```python
from build123d import *

# Parameters (mm, degrees)
F1_DEPTH = 5
F2_W     = 25
F2_H     = 5
F3_DEPTH = 15
F4_F1_R  = 5
F4_F2_R  = 4.9999


# Not quite as in the source:
# - a fillet or chamfer is up to 0.001 mm smaller than in the source, because OpenCascade refuses the exact size


with BuildPart() as f1:
    # F0 (on Front) → F1 (new body)
    with BuildSketch(Plane.XZ):
        with BuildLine():
            Line((-12.5, -22.5), (12.5, -22.5))
            Line((12.5, -22.5), (12.5, 22.5))
            Line((12.5, 22.5), (7.6, 22.5))
            ThreePointArc((7.6, 22.5), (0, 14.9), (-7.6, 22.5))
            Line((-7.6, 22.5), (-12.5, 22.5))
            Line((-12.5, 22.5), (-12.5, -22.5))
        make_face()
    extrude(amount=F1_DEPTH)

    # F2 (on face) → F3 (join)
    with BuildSketch(Plane.XZ.offset(5)):
        with Locations((0, -20)):
            Rectangle(F2_W, F2_H)
    extrude(amount=F3_DEPTH)

    # F4: fillet of radius 5 on 4 edges, made by hand

    # F4_f1
    f4_f1_edges = [f1.edges().sort_by_distance(p)[0] for p in [
        (0, -5, -17.5),
    ]]
    fillet(f4_f1_edges, radius=F4_F1_R)

    # F4_f2 (radius 5 in the source; OpenCascade refuses exactly that, so slightly less here)
    f4_f2_edges = [f1.edges().sort_by_distance(p)[0] for p in [
        (12.5, -15, -17.5),
        (-12.5, -15, -17.5),
        (0, -20, -17.5),
        (-12.5, -6.4644660941, -16.0355339059),
        (12.5, -6.4644660941, -16.0355339059),
    ]]
    fillet(f4_f2_edges, radius=F4_F2_R)


solid = f1.part
```
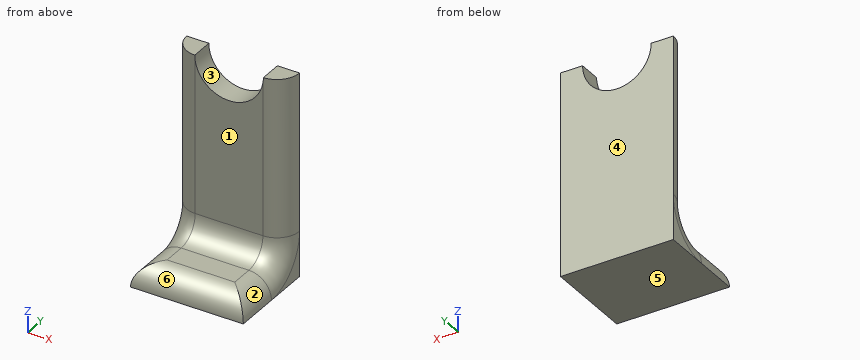
Geometry check sheet. Reference: the model listing, model coordinates, mm. Face numbers are marked on the shaded views. A direction names the side the tool comes from. Coordinates: 2 decimals unless noted, no trailing zeros. Answer in a Markdown table with one row per item. Add a question column.
1. Gauge pin test, flat ends, axial feed: pin 1 Ø5.5 at (x, y) = (2.5, -12) entering from +Z; pin 2 Ø6 at (x, z) = (-10, -8.5) entering from -Y; pin 3 Ø5 at (x, z) = (-9, -12.5) entering from -Y; pin 4 Ø2 at (x, z) = (3, -5.5) entering from +Y. Record the tip position at first contact, or that the pin passes through.
2. Draft check along Y on the marked faces 4, 5 and 6. Enter one of: +Y half, -Y half, draft (parallel to the pull), parting line (faces both ways), or undercut.
3. Access from +Z, -Z, +X, -X, +Y, -Y to the whole of each face (thin tool, end or side, straight path). Record for the marked faces 1, 2 and 3.
4. Material ranges on L1, parallel to Z at x = 3.75, y = -13.25; L2, parallel to Y at x = 6.5, z = 4; L3, parallel to X at y = -2.5, z = -7, recorded low to high. Write a range as [from, to].
Data:
| question | item | result |
|---|---|---|
| 1 | pin 1 | stops at z = -17.44 |
| 1 | pin 2 | stops at y = -5 |
| 1 | pin 3 | stops at y = -5.54 |
| 1 | pin 4 | stops at y = 0 |
| 2 | face 4 | +Y half |
| 2 | face 5 | draft |
| 2 | face 6 | -Y half |
| 3 | face 1 | +Z, +X, -X, -Y |
| 3 | face 2 | +Z, +X, -Y |
| 3 | face 3 | +Z, +Y, -Y |
| 4 | L1 | z = [-22.5, -17.5] |
| 4 | L2 | y = [-5, 0] |
| 4 | L3 | x = [-11.83, 11.83] |
